For this review, take the finished solid that the model builds, in its own axes (mm). Face numbers are marked on the shaded views. A direction names the side the tool comes from. Coordinates: 2 decimals unless noted, no trailing zeros. Order: outer loops, then holes, each group sorted by start corner. A loop starts at its lowest first (then second) coordinate and runs counter-clockwise, first axis right, second up. Notation, with made-up numbers: M 56,40.25 L 64,40.25 A28 ccw 64,73.25 Z; hole C 45.25,6.5 d8. An arc over 180 degrees is marked long. Use one line per item in the form item = value. Start each with the question number.
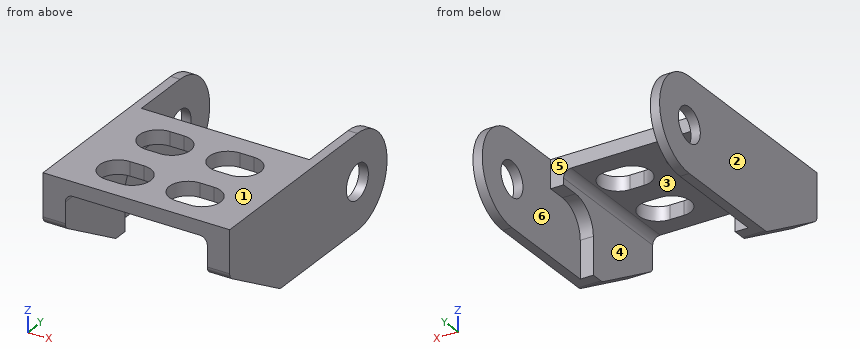
```python
from build123d import *

# Parameters (mm, degrees)
SKETCH1_W           = 20
SKETCH1_H           = 15
BOSS_EXTRUDE1_DEPTH = 1.5
SKETCH2_R           = 1.85
BOSS_EXTRUDE2_DEPTH = 2.4
CUT_EXTRUDE1_DEPTH  = 1.4
MIRROR1_START       = -10
MIRROR1_OUTLINE_R   = 1.85
MIRROR1_DEPTH       = 1
MIRROR1_START_2     = -9
MIRROR1_2_DEPTH     = 1.4
FILLET1_R           = 0.8
CUT_EXTRUDE2_DEPTH  = 1.5


# Read off the part's stored shape, not the designer's step: Mirror1
with BuildPart() as part:
    # Sketch1 → Boss-Extrude1 (new body)
    with BuildSketch(Plane.XY):
        Rectangle(SKETCH1_W, SKETCH1_H)
    extrude(amount=BOSS_EXTRUDE1_DEPTH)

    # Sketch2 → Boss-Extrude2 (add)
    with BuildSketch(Plane(origin=(10, 0, 0), x_dir=(0, 0, -1), z_dir=(1, 0, 0))):
        with BuildLine():
            Line((0, 7.5), (0, -7.5))
            Line((0, -7.5), (3.5, -7.5))
            Line((3.5, -7.5), (8.5, 1))
            Line((8.5, 1), (8.5, 14))
            ThreePointArc((8.5, 14), (3.5, 19), (-1.5, 14))
            Line((-1.5, 14), (-1.5, 7.5))
            Line((-1.5, 7.5), (0, 7.5))
        make_face()
        with Locations((3.5, 14)):
            Circle(SKETCH2_R, mode=Mode.SUBTRACT)
    extrude(amount=-BOSS_EXTRUDE2_DEPTH)

    # Sketch3 → Cut-Extrude1 (cut)
    with BuildSketch(Plane.ZY.offset(-7.6)):
        with BuildLine():
            Line((1.5, 7.5), (-1.5, 7.5))
            Line((-1.5, 7.5), (-1.5, 5.5))
            ThreePointArc((-1.5, 5.5), (-2.378679656, 3.378679656), (-4.5, 2.5))
            Line((-4.5, 2.5), (-8.5, 2.5))
            Line((-8.5, 2.5), (-8.5, 19.043681707))
            Line((-8.5, 19.043681707), (1.5, 19.043681707))
            Line((1.5, 19.043681707), (1.5, 7.5))
        make_face()
    extrude(amount=-CUT_EXTRUDE1_DEPTH, mode=Mode.SUBTRACT)

    # Mirror1 outline → Mirror1 (add)
    with BuildSketch(Plane.YZ.offset(MIRROR1_START)):
        with BuildLine():
            ThreePointArc((14, -8.5), (19, -3.5), (14, 1.5))
            Line((14, 1.5), (7.5, 1.5))
            Line((7.5, 1.5), (7.5, 0))
            Line((7.5, 0), (-7.5, 0))
            Line((-7.5, 0), (-7.5, -3.5))
            Line((-7.5, -3.5), (1, -8.5))
            Line((1, -8.5), (14, -8.5))
        make_face()
        with Locations((14, -3.5)):
            Circle(MIRROR1_OUTLINE_R, mode=Mode.SUBTRACT)
    extrude(amount=MIRROR1_DEPTH)

    # Mirror1 2 outline → Mirror1 2 (add)
    with BuildSketch(Plane.YZ.offset(MIRROR1_START_2)):
        with BuildLine():
            Line((1, -8.5), (2.5, -8.5))
            Line((2.5, -8.5), (2.5, -4.5))
            ThreePointArc((2.5, -4.5), (3.378679656, -2.378679656), (5.5, -1.5))
            Line((5.5, -1.5), (7.5, -1.5))
            Line((7.5, -1.5), (7.5, 0))
            Line((7.5, 0), (-7.5, 0))
            Line((-7.5, 0), (-7.5, -3.5))
            Line((-7.5, -3.5), (1, -8.5))
        make_face()
    extrude(amount=MIRROR1_2_DEPTH)

    # Fillet1
    fillet1_edges = [part.edges().sort_by_distance(p)[0] for p in [
        (8.8, 1, -8.5),
        (8.8, -7.5, -3.5),
        (7.6, 0, 0),
        (-8.8, 1, -8.5),
        (-7.6, 0, 0),
        (-8.8, -7.5, -3.5),
    ]]
    fillet(fillet1_edges, radius=FILLET1_R)

    # Sketch4 → Cut-Extrude2 (cut)
    with BuildSketch(Plane.XY.offset(1.5)):
        with BuildLine():
            Line((-4.5, 5.2), (-3, 5.2))
            ThreePointArc((-3, 5.2), (-1, 3.2), (-3, 1.2))
            Line((-3, 1.2), (-4.5, 1.2))
            ThreePointArc((-4.5, 1.2), (-6.5, 3.2), (-4.5, 5.2))
        make_face()
        with BuildLine():
            Line((3, 5.2), (4.5, 5.2))
            ThreePointArc((4.5, 5.2), (6.5, 3.2), (4.5, 1.2))
            Line((4.5, 1.2), (3, 1.2))
            ThreePointArc((3, 1.2), (1, 3.2), (3, 5.2))
        make_face()
        with BuildLine():
            Line((-4.5, -1.5), (-3, -1.5))
            ThreePointArc((-3, -1.5), (-1, -3.5), (-3, -5.5))
            Line((-3, -5.5), (-4.5, -5.5))
            ThreePointArc((-4.5, -5.5), (-6.5, -3.5), (-4.5, -1.5))
        make_face()
        with BuildLine():
            Line((3, -1.5), (4.5, -1.5))
            ThreePointArc((4.5, -1.5), (6.5, -3.5), (4.5, -5.5))
            Line((4.5, -5.5), (3, -5.5))
            ThreePointArc((3, -5.5), (1, -3.5), (3, -1.5))
        make_face()
    extrude(amount=-CUT_EXTRUDE2_DEPTH, mode=Mode.SUBTRACT)


solid = part.part
```
1. To check wall thickness, follow line 1 (X direction, y = 13, z = -6.5); line 2 (X direction, y = 1.25, z = -3.25); line 3 (Z direction, x = -9.65, y = 14). State the ranges of each line that lie inside material, in increasing order.
2. Consider section C-C, the plane y = -2.25. Write out the cut boundary in (x, z).
3. For pin 1 Ø1.1 at (x, y) = (-8, 6.5) entering from -Z; pin 2 Ø11 at (x, y) = (-1.5, 2.5) entering from -Z; pin 3 Ø1.2 at (x, z) = (4, 1) entering from +Y, all flat-tipped, find the tip position at first contact; note any pin that passes through.
4. Consider section A-A, the plane y = 9.5. Write out the cut boundary in (x, z).
5. Tool access review of the marked faces 4, 5 and 6: name each direction out of +Z, -Z, +X, -X, +Y, -Y from which nothing blocks a thin tool from reaching the whole face with its end or side.
6. Consider section D-D, the plane z = -5.75. Write out the cut boundary in (x, y) (3 decimals).
7. The part is to be moulded in two halves that separate along X. For the marked faces 1, 2 and 3, say which applies: pulls with the +X half, pulls with the -X half, needs draft (parallel to the pull), parting line crosses it, or undercut.
8. Consider section B-B, the plane x = 8. Write out the cut boundary in (y, z).
Answers follow:
q1.line_1 = -10 to -9, 9 to 10
q1.line_2 = -10 to -7.6, 7.6 to 10
q1.line_3 = -8.5 to -5.35, -1.65 to 1.5
q2.outline = M -10,-6.59 L -7.6,-6.59 L -7.6,-0.8 A0.8 cw -6.8,0 L -6.06,0 L -6.06,1.5 L -10,1.5 Z; M -1.44,0 L 1.44,0 L 1.44,1.5 L -1.44,1.5 Z; M 6.06,0 L 6.8,0 A0.8 cw 7.6,-0.8 L 7.6,-6.59 L 10,-6.59 L 10,1.5 L 6.06,1.5 Z
q3.pin_1 = -1.5
q3.pin_2 = -0.03
q3.pin_3 = 7.5
q4.outline = M -10,-8.5 L -9,-8.5 L -9,1.5 L -10,1.5 Z; M 9,-8.5 L 10,-8.5 L 10,1.5 L 9,1.5 Z
q5.face_4 = -Z, +Y, -Y
q5.face_5 = +Z, -Z, +Y
q5.face_6 = -Z, +Y
q6.outline = M -10,-3.675 L -7.6,-3.675 L -7.6,2.5 L -9,2.5 L -9,18.465 L -10,18.465 Z; M 7.6,-3.675 L 10,-3.675 L 10,18.465 L 9,18.465 L 9,2.5 L 7.6,2.5 Z
q7.face_1 = needs draft
q7.face_2 = pulls with the -X half
q7.face_3 = undercut
q8.outline = M -7.5,-3.04 A0.8 ccw -7.11,-3.73 L 0.81,-8.39 A0.8 ccw 1.22,-8.5 L 2.5,-8.5 L 2.5,-4.5 A3 cw 5.5,-1.5 L 7.5,-1.5 L 7.5,1.5 L -7.5,1.5 Z
